Could you check a few things on this model? Use its own coordinates, in mm. A direction names the side the tool comes from. Give positions to 0.01 mm unless a question says otherwise; leave off trailing zeros. Order: outer loops, then holes, each group sorted by start corner. A loop starts at its lowest first (then second) coordinate and runs counter-clockwise, first axis right, second up. Notation, with made-up numbers: (86, -39.5) -> (119, -39.5) arc R22 cw to (119, -31.5) -> close; hole circle Ø1 at (19.25, 33). An arc over 180 degrees is marked (long way). Write each question's results on one line, items separated by ' | '.
Autodesk Inventor part; units mm, degrees
ref_plane "YZ Plane" through (0, 0, 0) normal (1, 0, 0) x (0, 1, 0)
ref_plane "XZ Plane" through (0, 0, 0) normal (0, 1, 0) x (-1, 0, 0)
ref_plane "XY Plane" through (0, 0, 0) normal (0, 0, 1) x (1, 0, 0)
sketch "Sketch1" plane through (0, 0, 0) normal (0, 0, 1) x (1, 0, 0)
  circle A0 centre (0, 0) radius 2.5
  circle A1 centre (0, 0) radius 4
  dimension "d0" = 5
  dimension "d1" = 8
extrude "Extrusion1" add sketch "Sketch1" along normal blind 3.2
sketch "Sketch2" plane through (0, 0, 3.2) normal (0, 0, 1) x (1, 0, 0)
  circle A0 centre (0, 0) radius 2.5
extrude "Extrusion2" add sketch "Sketch2" against normal blind 1
sketch "Sketch3" plane through (0, 0, 3.2) normal (0, 0, 1) x (1, 0, 0)
  circle A0 centre (0, 0) radius 4
  circle A1 centre (0, 0) radius 2.5
  dimension "d6" = 5
extrude "Extrusion3" add sketch "Sketch3" along normal blind 1.6 contours A1
sketch "Sketch4" plane through (0, 0, 0) normal (0, 0, -1) x (-1, 0, 0)
  circle A0 centre (0, 0) radius 4
  circle A1 centre (0, 0) radius 3.25
  dimension "d9" = 6.5
extrude "Extrusion4" cut sketch "Sketch4" against normal blind 1.6
properties part number "4073" material "Steel"
Q1. For faces 1 (the cylindrical face through (2.579, -1.978, 0.789)), 2 (the flat face through (2, 2, 3.2)), 3 (the flat face through (2, -2, 0)), which set-ups out of +Z, -Z, +X, -X, +Y, -Y let a thin tool reach every point of the face, with its end or its side?
Here are the results:
face 1: -Z | face 2: +Z | face 3: -Z, +X, -X, +Y, -Y
Q2. Suppose I cut it at C-C on z = 1.05. Please give me the cut outline in (x, y).
Here are the results:
outline: circle Ø6.5 at (0, 0); hole circle Ø5 at (0, 0)
Q3. I need wall thicknesses on line 1 along Y through (x, z) = (0, 0.8); line 2 along Z through (x, y) = (1.5, 2.75); line 3 along Z through (x, y) = (3.25, 0.75). Which ranges of each line are inside material? Lowest first, please.
Here are the results:
line 1: y = -3.25 to -2.5, 2.5 to 3.25 | line 2: z = 0 to 3.2 | line 3: z = 1.6 to 3.2
Q4. I'm going to push flat-ended pins straight in: pin 1 Ø4 at (x, y) = (2, 1) entering from -Z; pin 2 Ø2.5 at (x, y) = (1, 0) entering from -Z. Where does each tip first touch, or does it pass through?
Here are the results:
pin 1: stops at z = 0 | pin 2: stops at z = 2.2
Q5. Suppose I cut it at D-D on z = 3.95. Please give me the cut outline in (x, y).
Here are the results:
outline: circle Ø5 at (0, 0)
Q6. Thinking about a two-plate mould opening in X: for faces 4 (the flat face through (0, 0, 2.2)), 5 (the flat face through (2, 3, 1.6)), 6 (the cylindrical face through (-0.54, 2.44, 3.99)), which applies, +X half, -X half, draft (parallel to the pull), parting line (faces both ways), or undercut?
Here are the results:
face 4: undercut | face 5: draft | face 6: parting line
Q7. Suppose I cut it at A-A on x = 0. Please give me the cut outline in (y, z), and give its area (3 significant figures).
Here are the results:
outline: (-4, 1.6) -> (-3.25, 1.6) -> (-3.25, 0) -> (-2.5, 0) -> (-2.5, 2.2) -> (2.5, 2.2) -> (2.5, 0) -> (3.25, 0) -> (3.25, 1.6) -> (4, 1.6) -> (4, 3.2) -> (2.5, 3.2) -> (2.5, 4.8) -> (-2.5, 4.8) -> (-2.5, 3.2) -> (-4, 3.2) -> close | area: 20.2 mm²
